from build123d import *

# Parameters (mm, degrees)
F1_DEPTH = 25.4
F2_DEPTH = 76.2
F3_R     = 12.7
F4_DEPTH = 127.001
F5_R     = 12.7
F6_DEPTH = 25.401


with BuildPart() as f1:
    # F0 (on Top) → F1 (new body)
    with BuildSketch(Plane.XY):
        Polygon((79.768824, 66.81983), (3.568824, 66.81983), (3.568824, 16.01983), (-21.831176, 16.01983), (-21.831176, -34.78017), (79.768824, -34.78017), align=None)
    extrude(amount=F1_DEPTH)

    # F0 (on Top) → F2 (join)
    with BuildSketch(Plane.XY):
        Polygon((79.768824, -110.98017), (79.768824, -34.78017), (-21.831176, -34.78017), (-21.831176, -60.18017), (54.368824, -60.18017), (54.368824, -110.98017), align=None)
    extrude(amount=F2_DEPTH)

    # F3 (on face) → F4 (cut, through all)
    with BuildSketch(Plane.XZ.offset(60.18017)):
        with Locations((16.268824, 50.8)):
            Circle(F3_R)
    extrude(amount=-F4_DEPTH, mode=Mode.SUBTRACT)

    # F5 (on face) → F6 (cut, through all)
    with BuildSketch(Plane.XY.offset(25.4)):
        with Locations((41.668824, 41.41983)):
            Circle(F5_R)
    extrude(amount=-F6_DEPTH, mode=Mode.SUBTRACT)


solid = f1.part
Part model, mm, in its own coordinate system. A direction names the side the tool comes from. Round coordinates to 2 decimals unless told otherwise and drop trailing zeros. Write each loop counter-clockwise with the first axis right and the second up, starting at its lowest first coordinate (ties: lowest second). Pieces come first, ordered by that corner, then holes. Notation, with made-up numbers: M 5,-39 L 49,-39 A27 ccw 49,-14 Z; hole C 52.5,4 d3. An arc over 180 degrees is marked long. Return JSON: item names as keys, results as strings. Group by question number.
(1) Pin check, flat tips, straight feed: pin 1 Ø8 at (x, z) = (5.5, 58) entering from +Y; pin 2 Ø4 at (x, z) = (30.5, 10) entering from -Y; pin 3 Ø20.5 at (y, z) = (46.5, 16) entering from -X. Stop position of each tip, or through.
(2) Two-plate mould, pull along X, no slides. Class faces 1 (the face through (3.569, 42, 13)), 2 (the face through (6.19, -47.66, 43.07)), 3 (the face through (15.7, -60.18, 37.6)): +X half, -X half, draft (parallel to the pull), parting line (faces both ways), or undercut.
(3) Saw through at D-D on x = 61. Write the cut outline in (y, z), then the cut area to 3 significant figures.
(4) Which spindle directions (+Z, -Z, +X, -X, +Y, -Y) get a long thin tool onto all of the face, cutting with end or side? Do faces 4 (the face through (67, -110.98, 38)), 5 (the face through (-9, 16.02, 13)), 6 (the face through (30, -34.78, 50)), 7 (the face through (54.369, -85, 38)). Say none if no direction does.
(5) Drill centre lines: probe 1 along Z at (x, y) = (6, -27); probe 2 along Y at (x, z) = (15.5, 66.5); probe 3 along Y at (x, z) = (57, 26.5). Where is each one in solid material? Low to high.
(6) Saw through at C-C on x = 36.5. Write the cut outline in (y, z).
(7) Saw through at A-A on z = 50.8. Write the cut outline in (x, y).
(8) Saw through at B-B on y = 36.5. Write the cut outline in (x, z).
Returned:
{
 "1": {"pin 1": "y = -34.78", "pin 2": "y = -60.18", "pin 3": "x = 3.57"},
 "2": {"face 1": "-X half", "face 2": "undercut", "face 3": "draft"},
 "3": {"outline": "M -110.98,0 L 66.82,0 L 66.82,25.4 L -34.78,25.4 L -34.78,76.2 L -110.98,76.2 Z", "area": "8,390 mm²"},
 "4": {"face 4": "+Z, -Z, +X, -X, -Y", "face 5": "+Z, -Z, -X, +Y", "face 6": "+Z, +X, -X, +Y", "face 7": "+Z, -Z, -X, -Y"},
 "5": {"probe 1": "0 to 25.4", "probe 2": "-60.18 to -34.78", "probe 3": "-110.98 to -34.78"},
 "6": {"outline": "M -60.18,0 L 29.82,0 L 29.82,25.4 L -34.78,25.4 L -34.78,76.2 L -60.18,76.2 Z; M 53.02,0 L 66.82,0 L 66.82,25.4 L 53.02,25.4 Z"},
 "7": {"outline": "M -21.83,-60.18 L 3.57,-60.18 L 3.57,-34.78 L -21.83,-34.78 Z; M 28.97,-60.18 L 54.37,-60.18 L 54.37,-110.98 L 79.77,-110.98 L 79.77,-34.78 L 28.97,-34.78 Z"},
 "8": {"outline": "M 3.57,0 L 29.96,0 L 29.96,25.4 L 3.57,25.4 Z; M 53.38,0 L 79.77,0 L 79.77,25.4 L 53.38,25.4 Z"}
}
